```python
from build123d import *

# Parameters (mm, degrees)
SKETCH1_R           = 35
SKETCH1_W           = 30
SKETCH1_H           = 20
BOSS_EXTRUDE1_DEPTH = 6.35
SKETCH2_W           = 6.35
SKETCH2_H           = 20
BOSS_EXTRUDE2_DEPTH = 20
SKETCH3_R           = 2.5
CUT_EXTRUDE1_DEPTH  = 57
FILLET1_R           = 10


with BuildPart() as part:
    # Sketch1 → Boss-Extrude1 (new body)
    with BuildSketch(Plane(origin=(0, 0, 0), x_dir=(1, 0, 0), z_dir=(0, 1, 0))):
        with Locations(Location((0, 0, 0), (0, 0, 270))):
            Circle(SKETCH1_R)
        Rectangle(SKETCH1_W, SKETCH1_H, mode=Mode.SUBTRACT)
    extrude(amount=BOSS_EXTRUDE1_DEPTH)

    # Sketch2 → Boss-Extrude2 (add)
    with BuildSketch(Plane(origin=(0, 6.35, 0), x_dir=(1, 0, 0), z_dir=(0, 1, 0))):
        with Locations((-18.175, 0)):
            Rectangle(SKETCH2_W, SKETCH2_H)
        with Locations((18.175, 0)):
            Rectangle(SKETCH2_W, SKETCH2_H)
    extrude(amount=BOSS_EXTRUDE2_DEPTH)

    # Sketch3 → Cut-Extrude1 (cut)
    with BuildSketch(Plane(origin=(21.35, 0, 0), x_dir=(0, 0, -1), z_dir=(1, 0, 0))):
        with Locations((0, 16.35)):
            Circle(SKETCH3_R)
    extrude(amount=-CUT_EXTRUDE1_DEPTH, mode=Mode.SUBTRACT)

    # Fillet1
    fillet1_edges = [part.edges().sort_by_distance(p)[0] for p in [
        (18.175, 26.35, -10),
        (18.175, 26.35, 10),
        (-18.175, 26.35, -10),
        (-18.175, 26.35, 10),
    ]]
    fillet(fillet1_edges, radius=FILLET1_R - 0.0001)  # a hair under: the kernel refuses the full size


solid = part.part
```
The model under review builds one solid part; all positions refer to its coordinate system, in mm. A direction names the side the tool comes from. Round coordinates to 2 decimals unless told otherwise and drop trailing zeros. Loops run counter-clockwise (first coordinate to the right, second up) from the corner with the lowest first, then second, coordinate; pieces in that order, holes last.
Item 1: For line 1 (X direction, y = 21, z = 5); line 2 (Y direction, x = -16.75, z = 0); line 3 (Y direction, x = 9, z = 15.5), list the stretches that pass through material, from the lowest coordinate up.
Determined:
line 1: x = -21.35 to -15, 15 to 21.35
line 2: y = 0 to 13.85, 18.85 to 26.35
line 3: y = 0 to 6.35
Item 2: Take a section at D-D (x = 27). Write out the cut boundary in (y, z).
Determined:
outline: (0, -22.27) - (6.35, -22.27) - (6.35, 22.27) - (0, 22.27) - close
Item 3: For faces 1 (the face through (-18, 11, -10)), 2 (the face through (21.35, 14, -2)), 3 (the face through (-21.35, 14, -2)), 4 (the face through (-15, 13, 0)), list the 3-axis set-ups (+Z, -Z, +X, -X, +Y, -Y) from which the entire face can be reached by the end or side of a thin tool; tool diameter is ignored.
Determined:
face 1: -Z, +X, -X, +Y
face 2: +Z, -Z, +X, +Y
face 3: +Z, -Z, -X, +Y
face 4: +Y, -Y
Item 4: Take a section at B-B (x = 0). Write out the cut boundary in (y, z), then the cut area to 4 significant figures.
Determined:
outline: (0, -35) - (6.35, -35) - (6.35, -10) - (0, -10) - close; (0, 10) - (6.35, 10) - (6.35, 35) - (0, 35) - close
area: 317.5 mm2
Item 5: Take a section at C-C (y = 3.75). Write out the cut boundary in (x, z).
Determined:
outline: circle Ø70 at (0, 0); hole (-15, -10) - (15, -10) - (15, 10) - (-15, 10) - close
Item 6: Take a section at A-A (y = 11.25). Write out the cut boundary in (x, z), then the cut area to 3 significant figures.
Determined:
outline: (-21.35, -10) - (-15, -10) - (-15, 10) - (-21.35, 10) - close; (15, -10) - (21.35, -10) - (21.35, 10) - (15, 10) - close
area: 254 mm2
Item 7: Clearance check with flat-ended pins moving along their axes: pin 1 Ø10 at (y, z) = (21, 1.5) entering from +X; pin 2 Ø12 at (x, z) = (-3.5, -21) entering from -Y; pin 3 Ø1.9 at (x, y) = (-17.5, 9.5) entering from +Z; pin 4 Ø1.9 at (x, y) = (-19, 13.5) entering from -Z. State where each tip first meets the part, or that it passes through.
Determined:
pin 1: stops at x = 21.35
pin 2: stops at y = 0
pin 3: stops at z = 10
pin 4: stops at z = -10
Item 8: Mouldability with a two-part tool opening along Y and no side actions: class faces 5 (the face through (0, 3, 10)), 6 (the face through (18.22, 18.46, -1.34)), 7 (the face through (-18.13, 18.46, -1.34)), 8 (the face through (-18.13, 23.5, -6.99)) as released by +Y, released by -Y, zero draft, split by the parting line, or undercut.
Determined:
face 5: zero draft
face 6: undercut
face 7: undercut
face 8: released by +Y
